Can you work these out from the model? Positions are in its coordinate system, mm. A direction names the side the tool comes from. Coordinates: 2 decimals unless noted, no trailing zeros. Order: outer loops, then holes, each group sorted by start corner. A loop starts at its lowest first (then second) coordinate and runs counter-clockwise, first axis right, second up. Notation, with made-up numbers: (85.25, -8) -> (100.25, -8) arc R13 ccw to (100.25, 9) -> close; hole circle Ø6 at (-19.75, 21.25). An arc over 180 degrees is marked (long way). Write item = value, one per line. Start each with the question number.
from build123d import *

# Parameters (mm, degrees)
SKETCH1_W               = 50.8
SKETCH1_H               = 939.8
BOSS_EXTRUDE1_DEPTH     = 12.7
SHELL1_T                = -1.5875
CUT_EXTRUDE1_DEPTH      = 471.757326018
CUT_EXTRUDE1_DEPTH_BACK = 471.757326018
SKETCH3_R               = 2.4892
CUT_EXTRUDE2_DEPTH      = 471.757326018
CUT_EXTRUDE2_DEPTH_BACK = 471.757326018
SKETCH4_R               = 3.175
SKETCH4_R_2             = 2.4892
SKETCH5_W               = 31.75
SKETCH5_H               = 26.9875
CUT_EXTRUDE3_DEPTH      = 471.757326018
FILLET1_R               = 3.175
CUT_EXTRUDE4_DEPTH      = 471.757326018
CUT_EXTRUDE4_DEPTH_BACK = 471.757326018
SKETCH6_R               = 3.175
SKETCH7_W               = 31.75
SKETCH7_H               = 26.9875
CUT_EXTRUDE5_DEPTH      = 471.757326018
FILLET2_R               = 3.175


with BuildPart() as part:
    # Sketch1 → Boss-Extrude1 (new, symmetric)
    with BuildSketch(Plane.XY):
        Rectangle(SKETCH1_W, SKETCH1_H)
    extrude(amount=BOSS_EXTRUDE1_DEPTH, both=True)

    # Shell1
    shell1_openings = [part.faces().sort_by_distance(p)[0] for p in [
        (0, -469.9, 0),
        (0, 469.9, 0),
    ]]
    offset(amount=SHELL1_T, openings=shell1_openings, kind=Kind.INTERSECTION)

    # Sketch3 → Cut-Extrude1 (cut, two sides: drawn at the far end of the back side and taken through both)
    with BuildSketch(Plane(origin=(0, 0, 0), x_dir=(0, 0, -1), z_dir=(1, 0, 0)).offset(-CUT_EXTRUDE1_DEPTH_BACK)):
        with Locations((0, -463.55)):
            Circle(SKETCH3_R)
        with Locations((0, -450.85)):
            Circle(SKETCH3_R)
    extrude(amount=CUT_EXTRUDE1_DEPTH + CUT_EXTRUDE1_DEPTH_BACK, mode=Mode.SUBTRACT)

    # Sketch4 → Cut-Extrude2 (cut, two sides: drawn at the far end of the back side and taken through both)
    with BuildSketch(Plane(origin=(0, 0, 0), x_dir=(0, 0, -1), z_dir=(1, 0, 0)).offset(-CUT_EXTRUDE2_DEPTH_BACK)):
        with Locations((-4.7625, -422.275)):
            Circle(SKETCH4_R)
        with Locations((-4.7625, -409.575)):
            Circle(SKETCH4_R_2)
        with Locations((-4.7625, -434.975)):
            Circle(SKETCH4_R_2)
    extrude(amount=CUT_EXTRUDE2_DEPTH + CUT_EXTRUDE2_DEPTH_BACK, mode=Mode.SUBTRACT)

    # Sketch5 → Cut-Extrude3 (cut, through all)
    with BuildSketch(Plane.XY):
        with Locations((0, -422.275)):
            Rectangle(SKETCH5_W, SKETCH5_H)
    extrude(amount=CUT_EXTRUDE3_DEPTH, mode=Mode.SUBTRACT)

    # Fillet1
    fillet1_edges = [part.edges().sort_by_distance(p)[0] for p in [
        (-15.875, -408.78125, 11.90625),
        (-15.875, -435.76875, 11.90625),
        (15.875, -435.76875, 11.90625),
        (15.875, -408.78125, 11.90625),
    ]]
    fillet(fillet1_edges, radius=FILLET1_R)

    # Sketch6 → Cut-Extrude4 (cut, two sides: drawn at the far end of the back side and taken through both)
    with BuildSketch(Plane(origin=(0, 0, 0), x_dir=(0, 0, -1), z_dir=(1, 0, 0)).offset(-CUT_EXTRUDE4_DEPTH_BACK)):
        with Locations((4.7625, 450.85)):
            Circle(SKETCH6_R)
    extrude(amount=CUT_EXTRUDE4_DEPTH + CUT_EXTRUDE4_DEPTH_BACK, mode=Mode.SUBTRACT)

    # Sketch7 → Cut-Extrude5 (cut, through all)
    with BuildSketch(Plane.XY):
        with Locations((0, 450.85)):
            Rectangle(SKETCH7_W, SKETCH7_H)
    extrude(amount=-CUT_EXTRUDE5_DEPTH, mode=Mode.SUBTRACT)

    # Fillet2
    fillet2_edges = [part.edges().sort_by_distance(p)[0] for p in [
        (15.875, 464.34375, -11.90625),
        (15.875, 437.35625, -11.90625),
        (-15.875, 437.35625, -11.90625),
        (-15.875, 464.34375, -11.90625),
    ]]
    fillet(fillet2_edges, radius=FILLET2_R)


solid = part.part
(1) Thinking about a two-plate mould opening in X: for faces 1 (the face through (0, 7, -11.112)), 2 (the face through (-25.4, -7, 0)), 3 (the face through (-23.812, -7, 0)), 4 (the face through (0, 469.9, -12)), which applies, +X half, -X half, draft (parallel to the pull), parting line (faces both ways), or undercut?
(2) Imagine slicing it at B-B (y = 338.5). Write out the boundary of the cut face in (x, z), plus the area to 3 significant figures.
(3) If I drill on L1, parallel to Y at x = -24.9, z = 0; L2, parallel to Z at x = -6.5, y = 96.5; L3, parallel to X at y = 184, z = -10.75, over which ranges is the centre line in solid material (lowest first)? Write a range as from..to.
(4) For P1, Ø12, axis at x = 16, z = 0, coming from the +Y side; P2, Ø8, axis at x = -15, z = -9, coming from the +Y side, each with a flat end and sliding along its axis, tell me the tip position at first contact or that it passes through.
(5) For faces 5 (the face through (0, -469.9, -12)), 6 (the face through (0, 7, 11.112)), which set-ups out of +Z, -Z, +X, -X, +Y, -Y let a thin tool reach every point of the face, with its end or its side?
(6) Imagine slicing it at A-A (x = 1). Write out the boundary of the cut face in (y, z), plus the area to 3 significant figures.
Result set:
q1.face_1 = undercut
q1.face_2 = -X half
q1.face_3 = undercut
q1.face_4 = draft
q2.outline = (-25.4, -12.7) -> (25.4, -12.7) -> (25.4, 12.7) -> (-25.4, 12.7) -> close; hole (-23.81, -11.11) -> (23.81, -11.11) -> (23.81, 11.11) -> (-23.81, 11.11) -> close
q2.area = 232 mm2
q3.L1 = -469.9..-466.04, -461.06..-453.34, -448.36..469.9
q3.L2 = -12.7..-11.11, 11.11..12.7
q3.L3 = -25.4..-23.81, 23.81..25.4
q4.P1 = through
q4.P2 = 469.9
q5.face_5 = +Z, -Z, +X, -X, -Y
q5.face_6 = +Y, -Y
q6.outline = (-469.9, -12.7) -> (437.36, -12.7) -> (437.36, -11.11) -> (-469.9, -11.11) -> close; (-469.9, 11.11) -> (-435.77, 11.11) -> (-435.77, 12.7) -> (-469.9, 12.7) -> close; (-408.78, 11.11) -> (469.9, 11.11) -> (469.9, 12.7) -> (-408.78, 12.7) -> close; (464.34, -12.7) -> (469.9, -12.7) -> (469.9, -11.11) -> (464.34, -11.11) -> close
q6.area = 2,900 mm2
